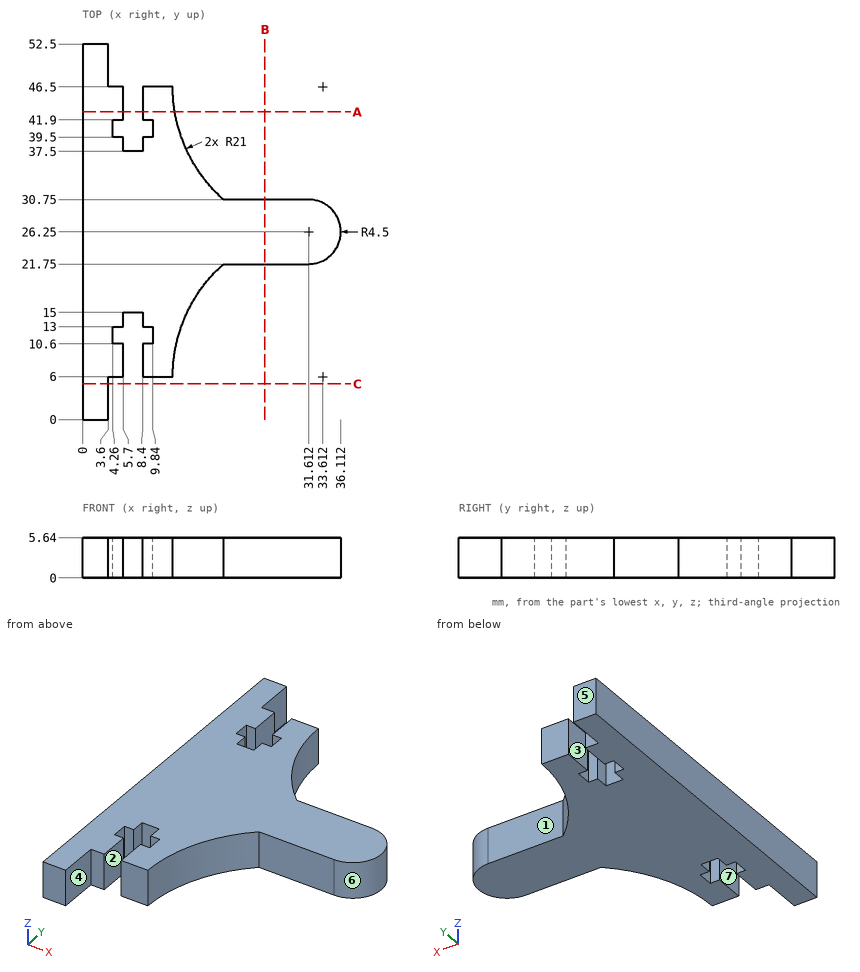
Verification items for this drawing (mm, ordinates from the low corner). A direction names the side the tool comes from. Coordinates: 2 decimals unless noted, no trailing zeros. Order: outer loops, then holes, each group sorted by start corner. A loop starts at its lowest first (then second) coordinate and runs counter-clockwise, first axis right, second up.
Q1. Tool access check on the marked faces 1, 2, 3 and 4. Record the directions out of +Z, -Z, +X, -X, +Y, -Y that give a thin tool (end or side, any length) a straight path to the whole face; none if there is none.
Reply:
face 1: +Z, -Z, +X, +Y
face 2: +Z, -Z, -Y
face 3: +Z, -Z, +Y
face 4: +Z, -Z, +X, -Y
Q2. Depth check by flat-ended pin: pin 1 Ø1.6 at (x, z) = (5, 2) entering from +Y; pin 2 Ø3 at (x, z) = (22.5, 2.5) entering from -Y; pin 3 Ø2 at (x, z) = (7, 2) entering from -Y. Enter the tip coordinate at first touch or a pass-through.
Reply:
pin 1: stops at y = 46.5
pin 2: stops at y = 21.75
pin 3: stops at y = 15
Q3. Draft check along X on the marked faces 5, 6 and 7. Enter one of: released by +X, released by -X, zero draft, split by the parting line, or undercut.
Reply:
face 5: zero draft
face 6: released by +X
face 7: undercut
Q4. Thickness scan on probe 1 along Y at (x, z) = (8.5, 4.2); probe 2 along Y at (x, z) = (22.5, 5.2); probe 3 along Y at (x, z) = (12.5, 1.7). Record the ranges inside material, lowest first.
Reply:
probe 1: y = 6 to 10.6, 13 to 39.5, 41.9 to 46.5
probe 2: y = 21.75 to 30.75
probe 3: y = 6 to 46.5
Q5. Sectioned sample at A-A on y = 43. Record the cut outline in (x, z) (1 decimal).
Reply:
outline: (0, 0) - (5.7, 0) - (5.7, 5.6) - (0, 5.6) - close; (8.4, 0) - (12.9, 0) - (12.9, 5.6) - (8.4, 5.6) - close
Q6. Sectioned sample at B-B on x = 25.5. Record the cut outline in (y, z).
Reply:
outline: (21.75, 0) - (30.75, 0) - (30.75, 5.64) - (21.75, 5.64) - close
Q7. Sectioned sample at C-C on y = 5. Record the cut outline in (x, z), and give its area (3 significant figures).
Reply:
outline: (0, 0) - (3.6, 0) - (3.6, 5.64) - (0, 5.64) - close
area: 20.3 mm2
